from build123d import *

# Parameters (mm, degrees)
SKETCH1_R                   = 17.4625
SKETCH1_R_2                 = 12.954
BOSS_EXTRUDE1_DEPTH         = 101.6
F_1_4_START                 = 12
F_1_4_CLEARANCE_SLOT1_DEPTH = 6
CUT_EXTRUDE1_REACH          = 106.558
CUT_EXTRUDE1_END_RADIUS     = 17.4625
CUT_EXTRUDE3_DEPTH          = 105.558298762
CUT_EXTRUDE3_DEPTH_BACK     = 105.558298762
SKETCH6_R                   = 3.3655
BOSS_EXTRUDE3_START         = 6.35
SKETCH8_R                   = 17.4625
BOSS_EXTRUDE3_DEPTH         = 6.35


with BuildPart() as part:
    # Sketch1 → Boss-Extrude1 (new body)
    with BuildSketch(Plane.XY):
        Circle(SKETCH1_R)
        Circle(SKETCH1_R_2, mode=Mode.SUBTRACT)
    extrude(amount=BOSS_EXTRUDE1_DEPTH)

    # 1/4 Clearance Slot1: read off the stored shape, not the designer's step
    # 1/4 Clearance Slot1 outline → 1/4 Clearance Slot1 (cut)
    with BuildSketch(Plane(origin=(0, 0, 0), x_dir=(1, 0, 0), z_dir=(0, 1, 0)).offset(F_1_4_START)):
        with BuildLine():
            Line((3.3782, -88.6968), (3.3782, -25.6032))
            ThreePointArc((3.3782, -25.6032), (0, -22.225), (-3.3782, -25.6032))
            Line((-3.3782, -25.6032), (-3.3782, -88.6968))
            ThreePointArc((-3.3782, -88.6968), (0, -92.075), (3.3782, -88.6968))
        make_face()
    extrude(amount=F_1_4_CLEARANCE_SLOT1_DEPTH, mode=Mode.SUBTRACT)

    # Cut-Extrude1: up to this cylinder (the profile starts inside it)
    cut_extrude1_end = Plane(origin=(0, 0, 57.15), z_dir=(0, 0, -1)) * Cylinder(CUT_EXTRUDE1_END_RADIUS, 249.041, mode=Mode.PRIVATE)
    # Sketch4 → Cut-Extrude1 (cut, up to the surface)
    with BuildSketch(Plane(origin=(0, 0, 0), x_dir=(1, 0, 0), z_dir=(0, 1, 0)), mode=Mode.PRIVATE) as cut_extrude1_sk1:
        with BuildLine():
            Line((-3.3782, -88.6968), (-3.3782, -25.6032))
            ThreePointArc((-3.3782, -25.6032), (0, -22.225), (3.3782, -25.6032))
            Line((3.3782, -25.6032), (3.3782, -88.6968))
            ThreePointArc((3.3782, -88.6968), (0, -92.075), (-3.3782, -88.6968))
        make_face()
    cut_extrude1_tool1 = extrude(cut_extrude1_sk1.sketch, amount=-CUT_EXTRUDE1_REACH, mode=Mode.PRIVATE) & cut_extrude1_end
    add(cut_extrude1_tool1.solids().sort_by_distance((0, 0, 57.15))[0], mode=Mode.SUBTRACT)

    # Sketch6 → Cut-Extrude3 (cut, two sides: drawn at the far end of the back side and taken through both)
    with BuildSketch(Plane(origin=(0, 0, 0), x_dir=(0, 0, -1), z_dir=(1, 0, 0)).offset(-CUT_EXTRUDE3_DEPTH_BACK)):
        with Locations((-9.525, 0)):
            Circle(SKETCH6_R)
    extrude(amount=CUT_EXTRUDE3_DEPTH + CUT_EXTRUDE3_DEPTH_BACK, mode=Mode.SUBTRACT)

    # Sketch8 → Boss-Extrude3 (add)
    with BuildSketch(Plane(origin=(0, 0, 0), x_dir=(-1, 0, 0), z_dir=(0, 0, -1)).offset(BOSS_EXTRUDE3_START)):
        Circle(SKETCH8_R)
    extrude(amount=-BOSS_EXTRUDE3_DEPTH)


solid = part.part
Could you check a few things on this model? Use its own coordinates, in mm. A direction names the side the tool comes from. Round coordinates to 2 decimals unless told otherwise and drop trailing zeros. Order: outer loops, then holes, each group sorted by start corner. A loop starts at its lowest first (then second) coordinate and runs counter-clockwise, first axis right, second up. Notation, with made-up numbers: M -14,-32.5 L 33,-32.5 A25 cw 33,-2.5 Z; hole C -19.75,76 d7. An arc over 180 degrees is marked long. One line per item, written item: value.
(1) Imagine slicing it at C-C (y = 0). Write out the boundary of the cut face in (x, z).
Ans:
outline: M -17.46,-6.35 L 17.46,-6.35 L 17.46,6.16 L 12.95,6.16 L 12.95,0 L -12.95,0 L -12.95,6.16 L -17.46,6.16 Z; M -17.46,12.89 L -12.95,12.89 L -12.95,101.6 L -17.46,101.6 Z; M 12.95,12.89 L 17.46,12.89 L 17.46,101.6 L 12.95,101.6 Z
(2) Imagine slicing it at B-B (x = 0). Count the separate pieces of the cut face and the enclosed holes in it, and give its area (3 significant figures).
Ans:
separate pieces: 3
enclosed holes: 0
area: 508 mm^2
(3) If we mould it in two halves opening along Z, with no side actions, what happens to faces 4 (the flat face through (0, 0, -6.35)), 5 (the flat face through (-3, 13, 101.6)), 6 (the cylindrical face through (-15.02, 2.27, 12.01))? For each: released by +Z, released by -Z, zero draft, split by the parting line, or undercut.
Ans:
face 4: released by -Z
face 5: released by +Z
face 6: undercut
(4) Imagine slicing it at D-D (z = 1). Write out the boundary of the cut face in (x, y) (1 decimal).
Ans:
outline: C 0,0 d34.9; hole C 0,0 d25.9
(5) I need wall thicknesses on line 1 along X through (y, z) = (0, 64.5); line 2 along Z through (x, y) = (16, 0); line 3 along X through (y, z) = (0.5, 43). Which ranges of each line are inside material? Lowest first, please. Write a range as from..to.
Ans:
line 1: x = -17.46..-12.95, 12.95..17.46
line 2: z = -6.35..6.16, 12.89..101.6
line 3: x = -17.46..-12.94, 12.94..17.46
(6) Which directions (+Z, -Z, +X, -X, +Y, -Y) give clear straight access to the entire face, cutting with the end or side of a thin tool? Please do faces 1 (the cylindrical face through (11.966, -4.961, 50.089)), 2 (the cylindrical face through (14.951, 1.011, 6.315)), 3 (the flat face through (-3.378, 15, 57)).
Ans:
face 1: +Z
face 2: +X, -X
face 3: +Y, -Y
(7) Imagine slicing it at A-A (z = 33.5). Write out the boundary of the cut face in (x, y) (1 decimal).
Ans:
outline: M -3.4,-17.1 L -3.4,-12.5 A13 cw -3.4,12.5 L -3.4,17.1 A17.5 ccw Z; M 3.4,-17.1 A17.5 ccw 3.4,17.1 L 3.4,12.5 A13 cw 3.4,-12.5 Z
(8) I'm going to push flat-ended pins straight in: P1, Ø2, axis at x = -10.5, z = 47.5, coming from the -Y side; P2, Ø13, axis at x = 3, y = -1, coming from the +Z side; P3, Ø2, axis at x = -13.5, z = 50, coming from the -Y side; P4, Ø4, axis at y = 0, z = 9.525, coming from the -X side. Where does each tip first touch, or does it pass through?
Ans:
P1: stops at y = -14.65
P2: stops at z = 0
P3: stops at y = -12.19
P4: passes through
